The model under review builds one solid part; all positions refer to its coordinate system, in mm. Face numbers are marked on the shaded views. A direction names the side the tool comes from. Coordinates: 2 decimals unless noted, no trailing zeros.
1) For line 1 (Y direction, x = 0, z = -133); line 2 (X direction, y = 6.5, z = -165); line 3 (Y direction, x = -2, z = -167), list the stretches that pass through material, from the lowest coordinate up.
2) For P1, Ø18, axis at x = 0, y = 0, coming from the +Z side; P2, Ø1, axis at y = 10.5, z = -39.5, coming from the -X side; P3, Ø22, axis at x = 2, y = -4, coming from the -Z side; P4, Ø10, axis at y = 25.5, z = -85, coming from the -X side, all flat-tipped, find the tip position at first contact; note any pin that passes through.
3) Machinability: for the marked faces 1 and 2, which of the approach directions +Z, -Z, +X, -X, +Y, -Y give a long, thin tool a straight path to every point of the face, cutting with its end or side? Answer none if there is none.
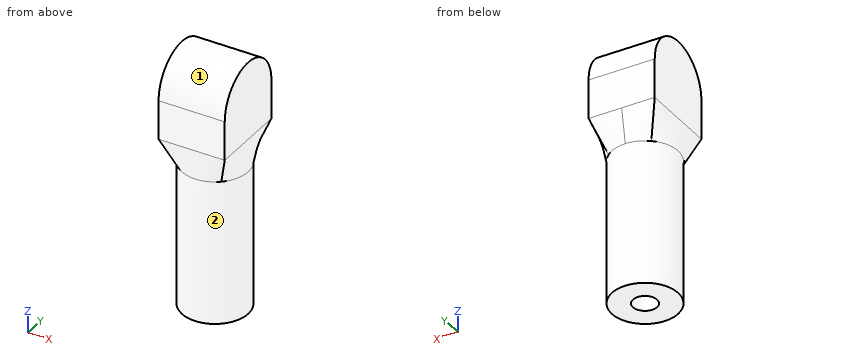
Autodesk Inventor part; units mm, degrees
ref_plane "Work Plane2" through (0, -32.5, -60) normal (0, 0, -1) x (0, 1, 0)
ref_plane "Work Plane1" through (0, 0, 27.5) normal (0, 0, 1) x (1, 0, 0)
ref_plane "Work Plane3" through (0, 0, -180) normal (0, 0, -1) x (-1, 0, 0)
sketch "Sketch6" plane through (0, 0, 0) normal (1, 0, 0) x (0, 1, 0)
  circle A0 centre (0, 0) radius 32.5
  line L0 (-32.5, 0) -> (-32.5, -60)
  line L1 (-32.5, -60) -> (32.5, -60)
  line L2 (32.5, -60) -> (32.5, 0)
  line L3 (0, 0) -> (0, -60) construction
  line L4 (-32.5, -32.5) -> (32.5, -32.5)
  dimension "d38" = 65
  dimension "d39" = 60
extrude "Extrusion8" add sketch "Sketch6" along normal mid plane 55 contours A0 | L2 L4 A0 | A0 L4 L0
ref_plane "Work Plane2" through (0, -32.5, -60) normal (0, 0, -1) x (0, 1, 0)
ref_plane "Work Plane1" through (0, 0, 27.5) normal (0, 0, 1) x (1, 0, 0)
sketch "Sketch3" plane through (0, -32.5, -60) normal (0, 0, -1) x (0, 1, 0)
  circle A0 centre (32.5, 0) radius 27.5
  line L0 (65, -27.5) -> (65, 27.5)
  circle A1 centre (32.5, 0) radius 37.5
  dimension "d48" = 10
  dimension "d73" = 55
loft "Loft1" add profiles "Sketch3" section 1 edges at (0, 32.5, -32.5) (27.5, 0, -32.5) (0, -32.5, -32.5) (-27.5, 0, -32.5) contours A0
sketch "Sketch7" plane through (0, 0, 0) normal (1, 0, 0) x (0, 1, 0)
  line L0 (20.9931, -60) -> (-20.9931, -60)
  line L1 (0, -60) -> (0, -180)
  point P0 (0, 0)
  dimension "d52" = 120
ref_plane "Work Plane3" through (0, 0, -180) normal (0, 0, -1) x (-1, 0, 0)
extrude "Extrusion1" add sketch "Sketch3" along normal blind 120 contours A0
sketch "Sketch5" plane through (0, 0, -180) normal (0, 0, -1) x (-1, 0, 0)
  circle A0 centre (0, 0) radius 10
  point P0 (0, 0)
  dimension "d35" = 20
extrude "Extrusion7" cut sketch "Sketch5" against normal blind 60
properties part number "shank_2"
Geometry results:
1. line 1: y = -27.5 to -10, 10 to 27.5
1. line 2: x = -26.72 to -7.6, 7.6 to 26.72
1. line 3: y = -27.43 to -9.8, 9.8 to 27.43
2. P1: stops at z = 32.5
2. P2: stops at x = -27.22
2. P3: stops at z = -180
2. P4: stops at x = -18.33
3. face 1: +Z, +X, -X
3. face 2: -Z
